Source: CAD feature listing. Evaluate the final solid. Frame: model axes, mm. Coordinates: 2 decimals unless noted, no trailing zeros. Order: outer loops, then holes, each group sorted by start corner. A loop starts at its lowest first (then second) coordinate and runs counter-clockwise, first axis right, second up. Notation, with made-up numbers: (31.25, -25.5) -> (59.25, -25.5) arc R24 ccw to (59.25, -3.5) -> close; hole circle Ø9 at (-20.5, 66). An arc over 180 degrees is marked (long way). Put each result on its own line as item: value.
from build123d import *

# Parameters (mm, degrees)
F2_DEPTH = 12.7
F4_D     = 6.35


# Not quite as in the source:
# - a variable given as a bare number and used for a length is read in inches; the dataset says mm whatever the document's units were


with BuildPart() as f2:
    # F1 (on Front) → F2 (new body)
    with BuildSketch(Plane.XZ):
        with BuildLine():
            Line((-25.4, 8.4416426996), (-25.4, 0))
            Line((-25.4, 0), (-12.7, 0))
            ThreePointArc((-12.7, 0), (-9.525, 3.175), (-6.35, 0))
            Line((-6.35, 0), (-3.175, 0))
            ThreePointArc((-3.175, 0), (0, 3.175), (3.175, 0))
            Line((3.175, 0), (6.35, 0))
            ThreePointArc((6.35, 0), (9.525, 3.175), (12.7, 0))
            Line((12.7, 0), (25.4, 0))
            Line((25.4, 0), (25.4, 8.4416426996))
            Line((25.4, 8.4416426996), (-25.4, 8.4416426996))
        make_face()
    extrude(amount=F2_DEPTH)

    # F4 (through all)
    with Locations(Plane.XY.offset(8.4416426996)):
        with Locations((-19.05, -6.35), (19.05, -6.35)):
            Hole(F4_D / 2)


solid = f2.part
1. Pull-direction query (Y, two-part tool) for faces 1 (the flat face through (0, 0, 4)), 2 (the cylindrical face through (-0.07, -6.261, 3.174)), 3 (the cylindrical face through (-15.88, -6.21, 4.16)); classes: pulls with the +Y half, pulls with the -Y half, needs draft (parallel to the pull), parting line crosses it, or undercut.
Numbers:
face 1: pulls with the +Y half
face 2: needs draft
face 3: undercut
2. Cut plane D-D on y = -11.5. Output: boundary loops of the cut face in (x, z) (3 decimals), plus the area to 3 significant figures.
Numbers:
outline: (-25.4, 0) -> (-12.7, 0) arc R3.175 cw to (-6.35, 0) -> (-3.175, 0) arc R3.175 cw to (3.175, 0) -> (6.35, 0) arc R3.175 cw to (12.7, 0) -> (25.4, 0) -> (25.4, 8.442) -> (-25.4, 8.442) -> close
area: 381 mm2
3. First-contact query: pin 1 (5 mm diameter, centred on x = 9.5, z = 6.5, fed in from +Y). Flat tip, straight axial feed; report the tip coordinate or a pass-through.
Numbers:
pin 1: stops at y = 0
4. Cut plane B-B on z = 1.75. Output: boundary loops of the cut face in (x, y) (3 decimals).
Numbers:
outline: (-25.4, -12.7) -> (-12.174, -12.7) -> (-12.174, 0) -> (-25.4, 0) -> close; (-6.876, -12.7) -> (-2.649, -12.7) -> (-2.649, 0) -> (-6.876, 0) -> close; (2.649, -12.7) -> (6.876, -12.7) -> (6.876, 0) -> (2.649, 0) -> close; (12.174, -12.7) -> (25.4, -12.7) -> (25.4, 0) -> (12.174, 0) -> close; hole circle Ø6.35 at (-19.05, -6.35); hole circle Ø6.35 at (19.05, -6.35)
5. Cut plane C-C on y = -5.25. Output: boundary loops of the cut face in (x, z) (3 decimals), plus the area to 3 significant figures.
Numbers:
outline: (-25.4, 0) -> (-22.028, 0) -> (-22.028, 8.442) -> (-25.4, 8.442) -> close; (-16.072, 0) -> (-12.7, 0) arc R3.175 cw to (-6.35, 0) -> (-3.175, 0) arc R3.175 cw to (3.175, 0) -> (6.35, 0) arc R3.175 cw to (12.7, 0) -> (16.072, 0) -> (16.072, 8.442) -> (-16.072, 8.442) -> close; (22.028, 0) -> (25.4, 0) -> (25.4, 8.442) -> (22.028, 8.442) -> close
area: 281 mm2
6. Cut plane A-A on x = 19.05. Output: boundary loops of the cut face in (y, z) (3 decimals), plus the area to 3 significant figures.
Numbers:
outline: (-12.7, 0) -> (-9.525, 0) -> (-9.525, 8.442) -> (-12.7, 8.442) -> close; (-3.175, 0) -> (0, 0) -> (0, 8.442) -> (-3.175, 8.442) -> close
area: 53.6 mm2
7. Ray query, line 1 along X through (y, z) = (-6.25, 5); line 2 along Y through (x, z) = (-19.05, 5.5) (3 decimals); line 3 along X through (y, z) = (-5.5, 6.25). Return the intervals inside material, ascending.
Numbers:
line 1: x = -25.4 to -22.22, -15.88 to 15.88, 22.22 to 25.4
line 2: y = -12.7 to -9.525, -3.175 to 0
line 3: x = -25.4 to -22.11, -15.99 to 15.99, 22.11 to 25.4
